```python
from build123d import *

# Parameters (mm, degrees)
F1_DEPTH = 82.042
F2_SIZE  = 50.8


with BuildPart() as f1:
    # F0 (on Front) → F1 (new body)
    with BuildSketch(Plane.XZ):
        Polygon((16.948685, 57.259064), (-44.738416, 33.439294), (-37.714638, -25.193989), (32.217763, -14.200249), align=None)
    extrude(amount=F1_DEPTH)

    # F2
    f2_edges = [f1.edges().sort_by_distance(p)[0] for p in [
        (16.948685, -41.021, 57.259064),
    ]]
    chamfer(f2_edges, length=F2_SIZE)


solid = f1.part
```
For this review, take the finished solid that the model builds, in its own axes (mm). Coordinates: 2 decimals unless noted, no trailing zeros. Write each loop counter-clockwise with the first axis right and the second up, starting at its lowest first coordinate (ties: lowest second). Pieces come first, ordered by that corner, then holes. Notation, with made-up numbers: (11, -34.75) - (37, -34.75) arc R5 ccw to (37, -29.75) - close; hole circle Ø2 at (12, 51). An arc over 180 degrees is marked (long way). Answer in a Markdown table with one row per item. Add a question column.
Q1. For P1, Ø3, axis at x = 0, y = -60.5, coming from the -Z side; P2, Ø2, axis at y = -71.5, z = 9.5, coming from the -X side; P3, Ø6, axis at y = -59.5, z = 29.5, coming from the -X side, all flat-tipped, find the tip position at first contact; note any pin that passes through.
Q2. For probe 1 along Z at (x, y) = (-2, -30); probe 2 along X at (y, z) = (-43, 27.5); probe 3 along X at (y, z) = (-28, 14), list the stretches that pass through material, from the lowest coordinate up.
Q3. We need section B-B, the plane x = -17. State the section outline as (y, z) points, and give its area (3 significant figures).
Q4. We need section C-C, the plane z = 30. State the section outline as (x, y) points.
Q5. We need section A-A, the plane y = -60. State the section outline as (x, z) points, and give its area (3 significant figures).
Answer list:
| question | item | result |
|---|---|---|
| 1 | P1 | stops at z = -19.5 |
| 1 | P2 | stops at x = -41.99 |
| 1 | P3 | stops at x = -44.63 |
| 2 | probe 1 | z = -19.58 to 23.57 |
| 2 | probe 2 | x = -44.03 to -9.26 |
| 2 | probe 3 | x = -42.41 to 15.7 |
| 3 | outline | (-82.04, -21.94) - (0, -21.94) - (0, 31.69) - (-82.04, 31.69) - close |
| 3 | area | 4,400 mm2 |
| 4 | outline | (-44.33, -82.04) - (-13.88, -82.04) - (-13.88, 0) - (-44.33, 0) - close |
| 5 | outline | (-44.74, 33.44) - (-37.71, -25.19) - (32.22, -14.2) - (27.56, 7.58) - (-30.44, 38.96) - close |
| 5 | area | 3,200 mm2 |
